Source: CAD feature listing. Evaluate the final solid. Frame: model axes, mm. Face numbers are marked on the shaded views. Coordinates: 2 decimals unless noted, no trailing zeros. Loops run counter-clockwise (first coordinate to the right, second up) from the corner with the lowest first, then second, coordinate; pieces in that order, holes last. Notation, with made-up numbers: M -22.5,28 L 13.5,28 A19 ccw 13.5,40 Z; hole C 58,71 d2. An arc over 180 degrees is marked long. Write each question's results on one line, items separated by ' | '. Start each with the question number.
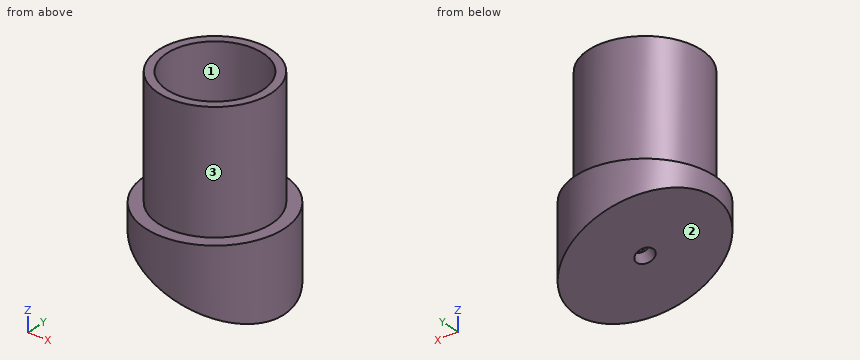
from build123d import *

# Parameters (mm, degrees)
SKETCH2_R               = 13.25
BOSS_EXTRUDE1_DEPTH     = 28
SKETCH3_R               = 16.25
BOSS_EXTRUDE2_DEPTH     = 28
CUT_EXTRUDE1_DEPTH      = 61.532016322
CUT_EXTRUDE1_DEPTH_BACK = 61.532016322
CUT_EXTRUDE2_REACH      = 53.777
SKETCH5_R               = 11.25
SKETCH6_R               = 2.1
CUT_EXTRUDE3_DEPTH      = 5
CUT_EXTRUDE4_DEPTH      = 2


with BuildPart() as part:
    # Sketch2 → Boss-Extrude1 (new body)
    with BuildSketch(Plane.XY):
        Circle(SKETCH2_R)
    extrude(amount=-BOSS_EXTRUDE1_DEPTH)

    # Sketch3 → Boss-Extrude2 (add)
    with BuildSketch(Plane(origin=(0, 0, -28), x_dir=(-1, 0, 0), z_dir=(0, 0, -1))):
        Circle(SKETCH3_R)
    extrude(amount=BOSS_EXTRUDE2_DEPTH)

    # Sketch4 → Cut-Extrude1 (cut, two sides: drawn at the far end of the back side and taken through both)
    with BuildSketch(Plane(origin=(0, 0, 0), x_dir=(1, 0, 0), z_dir=(0, 1, 0)).offset(-CUT_EXTRUDE1_DEPTH_BACK)):
        Polygon((-16.25, 32.602284237), (16.25, 46.397715763), (16.25, 56), (-16.25, 56), align=None)
    extrude(amount=CUT_EXTRUDE1_DEPTH + CUT_EXTRUDE1_DEPTH_BACK, mode=Mode.SUBTRACT)

    # Cut-Extrude2: up to this plane
    cut_extrude2_end = Plane(origin=(-14.296344358, -16.25, -27.999759969), z_dir=(0.3907311284892747, 0, 0.9205048534524399))
    # Sketch5 → Cut-Extrude2 (cut, up to the surface)
    with BuildSketch(Plane.XY, mode=Mode.PRIVATE) as cut_extrude2_sk1:
        Circle(SKETCH5_R)
    cut_extrude2_tool1 = split(extrude(cut_extrude2_sk1.sketch, amount=-CUT_EXTRUDE2_REACH, mode=Mode.PRIVATE), bisect_by=cut_extrude2_end, keep=Keep.BOTH, mode=Mode.PRIVATE)
    add(cut_extrude2_tool1.solids().sort_by_distance((0, 0, 0))[0], mode=Mode.SUBTRACT)

    # Sketch6 → Cut-Extrude3 (cut)
    with BuildSketch(Plane(origin=(-14.206961057, 0, -33.469502817), x_dir=(-0.9205048534524399, 0, 0.3907311284892748), z_dir=(-0.3907311284892748, 0, -0.9205048534524399))):
        with Locations((-15.433879575, 0)):
            Circle(SKETCH6_R)
    extrude(amount=-CUT_EXTRUDE3_DEPTH, mode=Mode.SUBTRACT)

    # Sketch7 → Cut-Extrude4 (cut)
    with BuildSketch(Plane(origin=(-12.253305414, 0, -28.866978549), x_dir=(0.9205048534524399, 0, -0.3907311284892748), z_dir=(0.3907311284892748, 0, 0.9205048534524399))):
        Polygon((19.533879575, 0), (17.483879575, 3.550704156), (13.383879575, 3.550704156), (11.333879575, 0), (13.383879575, -3.550704156), (17.483879575, -3.550704156), align=None)
    extrude(amount=-CUT_EXTRUDE4_DEPTH, mode=Mode.SUBTRACT)


solid = part.part
Item 1: Cut plane A-A (z = -14.5). Output: boundary loops of the cut face in (x, y), then the cut area to 3 significant figures.
Item 2: Mould query, pull axis X, two halves, no side actions, for the marked faces 1, 2 and 3. Classes: +X half, -X half, draft (parallel to the pull), parting line (faces both ways), or undercut.
Item 3: First-contact query: pin 1 Ø1.7 at (x, z) = (2.5, -36.5) entering from +Y; pin 2 Ø5 at (x, y) = (5, -2) entering from -Z; pin 3 Ø2 at (x, z) = (12.5, -19) entering from -Y. Flat tips, straight axial feed; report the tip coordinate or a pass-through.
Item 4: Cut plane C-C (x = -7.5). Output: boundary loops of the cut face in (y, z), then the cut area to 3 significant figures.
Item 5: Cut plane B-B (y = -6). Output: boundary loops of the cut face in (x, z).
Item 6: Line query: probe 1 along Y at (x, z) = (0, -16); probe 2 along Y at (x, z) = (0, -31); probe 3 along X at (y, z) = (-2, -12). Output: solid intervals per line, ascending.
Item 7: Cut plane D-D (z = -32). Output: boundary loops of the cut face in (x, y), then the cut area to 3 significant figures.
Response values:
1) outline: C 0,0 d26.5; hole C 0,0 d22.5 | area: 154 mm2
2) face 1: undercut | face 2: -X half | face 3: parting line
3) pin 1: stops at y = 16.17 | pin 2: stops at z = -42.68 | pin 3: stops at y = -6.58
4) outline: M -14.42,-36.32 L 14.42,-36.32 L 14.42,-28 L 10.92,-28 L 10.92,0 L 8.39,0 L 8.39,-30.88 L -8.39,-30.88 L -8.39,0 L -10.92,0 L -10.92,-28 L -14.42,-28 Z | area: 334 mm2
5) outline: M -15.1,-33.09 L 15.1,-45.91 L 15.1,-28 L 11.81,-28 L 11.81,0 L 9.52,0 L 9.52,-38.11 L -9.52,-30.03 L -9.52,0 L -11.81,0 L -11.81,-28 L -15.1,-28 Z
6) probe 1: y = -13.25 to -11.25, 11.25 to 13.25 | probe 2: y = -16.25 to -11.25, 11.25 to 16.25 | probe 3: x = -13.1 to -11.07, 11.07 to 13.1
7) outline: C 0,0 d32.5; hole M -4.87,-10.14 A11.25 ccw long -4.87,10.14 Z | area: 525 mm2
